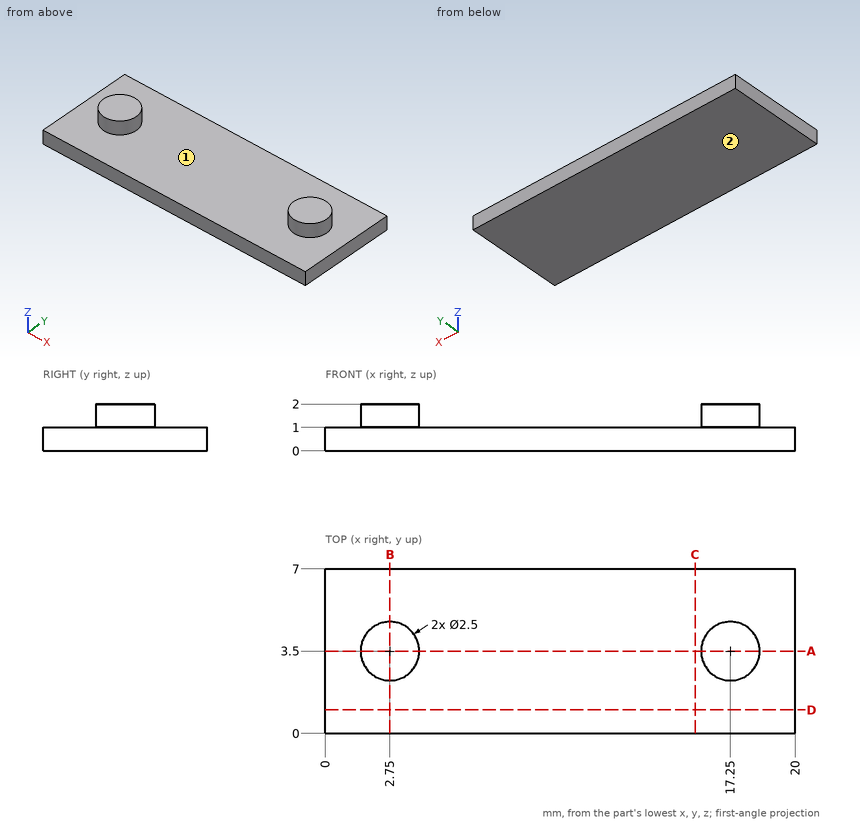
Here's the drawing with two shaded views (mm, measured from the low corner). I have some questions. Coordinates: 2 decimals unless noted, no trailing zeros. Loops run counter-clockwise (first coordinate to the right, second up) from the corner with the lowest first, then second, coordinate; pieces in that order, holes last. Notation, with made-up numbers: (29.5, 80.5) - (82.5, 80.5) arc R19 cw to (82.5, 102.5) - close; hole circle Ø11 at (30.5, 69). An arc over 180 degrees is marked (long way). Answer as CSV lines item,"result". Start each with the question number.
1) Thinking about a two-plate mould opening in X: for the marked faces 1 and 2, which applies, pulls with the +X half, pulls with the -X half, needs draft (parallel to the pull), parting line crosses it, or undercut?
2) Suppose I cut it at A-A (y = 3.5). Please give me the cut outline in (x, z).
3) I need wall thicknesses on line 1 (Z direction, x = 1, y = 5.75); line 2 (X direction, y = 3, z = 1.3). Which ranges of each line are inside material? Lowest first, please. Write a range as from..to.
4) Suppose I cut it at B-B (x = 2.75). Please give me the cut outline in (y, z).
5) Suppose I cut it at C-C (x = 15.75). Please give me the cut outline in (y, z), plus the area to 3 significant figures.
6) Suppose I cut it at D-D (y = 1). Please give me the cut outline in (x, z), plus the area to 3 significant figures.
Check result:
1,face 1,"undercut"
1,face 2,"needs draft"
2,outline,"(0, 0) - (20, 0) - (20, 1) - (18.5, 1) - (18.5, 2) - (16, 2) - (16, 1) - (4, 1) - (4, 2) - (1.5, 2) - (1.5, 1) - (0, 1) - close"
3,line 1,"z = 0..1"
3,line 2,"x = 1.6..3.9, 16.1..18.4"
4,outline,"(0, 0) - (7, 0) - (7, 1) - (4.75, 1) - (4.75, 2) - (2.25, 2) - (2.25, 1) - (0, 1) - close"
5,outline,"(0, 0) - (7, 0) - (7, 1) - (0, 1) - close"
5,area,"7.00 mm²"
6,outline,"(0, 0) - (20, 0) - (20, 1) - (0, 1) - close"
6,area,"20.0 mm²"
